The model under review builds one solid part; all positions refer to its coordinate system, in mm. Coordinates: 2 decimals unless noted, no trailing zeros. Write each loop counter-clockwise with the first axis right and the second up, starting at its lowest first coordinate (ties: lowest second). Pieces come first, ordered by that corner, then holes.
1) Add section B-B, the plane z = -60. State the section outline as (x, y) points.
2) For line 1 (Z direction, x = -60, y = -1.85); line 2 (Z direction, x = -37.5, y = -2.9), list the stretches that pass through material, from the lowest coordinate up.
3) Add section A-A, the plane x = -60. State the section outline as (y, z) points.
4) For P1, Ø8, axis at x = 54.5, z = -30.5, coming from the +Y side, flat-tipped, find the tip position at first contact; note if it passes through.
from build123d import *

# Parameters (mm, degrees)
F0_W     = 150
F0_H     = 150
F0_R     = 5.5
F0_W_2   = 19
F0_H_2   = 12
F1_DEPTH = 3


with BuildPart() as f1:
    # F0 (on Front) → F1 (new body)
    with BuildSketch(Plane.XZ):
        Rectangle(F0_W, F0_H)
        with Locations((-60, -60)):
            Circle(F0_R, mode=Mode.SUBTRACT)
        with Locations((-35.5, -60)):
            Rectangle(F0_W_2, F0_H_2, mode=Mode.SUBTRACT)
    extrude(amount=F1_DEPTH)


solid = f1.part
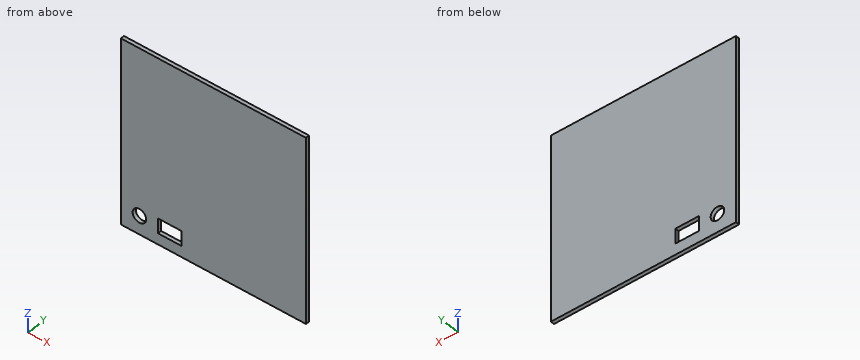
Geometry results:
1. outline: (-75, -3) - (-65.5, -3) - (-65.5, 0) - (-75, 0) - close; (-54.5, -3) - (-45, -3) - (-45, 0) - (-54.5, 0) - close; (-26, -3) - (75, -3) - (75, 0) - (-26, 0) - close
2. line 1: z = -75 to -65.5, -54.5 to 75
2. line 2: z = -75 to -66, -54 to 75
3. outline: (-3, -75) - (0, -75) - (0, -65.5) - (-3, -65.5) - close; (-3, -54.5) - (0, -54.5) - (0, 75) - (-3, 75) - close
4. P1: stops at y = 0
